CAD build for the part. Positions are in the model's coordinates, mm. A direction names the side the tool comes from. Round coordinates to 2 decimals unless told otherwise and drop trailing zeros. Write each loop counter-clockwise with the first axis right and the second up, starting at its lowest first coordinate (ties: lowest second). Pieces come first, ordered by that corner, then holes. Notation, with made-up numbers: (32, -10) - (36, -10) arc R30 cw to (36, 21) - close; hole circle Ø7 at (20.25, -36.75). An arc over 180 degrees is marked (long way). Put each result on its own line as item: value. Start each with the question number.
Item 1: Cut at B-B (z = 6). Give the cut face in (x, y).
Item 2: 3-axis set-ups, long thin cutter, end or side, ignore diameter. For faces 1 (the cylindrical face through (-2.579, -1.978, -0.493)), 2 (the flat face through (0, 0, -11)), 3 (the cylindrical face through (-0.325, -34.86, 4.536)), 4 (the flat face through (2, -2, 16)), 5 (the flat face through (0, -45, 6)): which of +Z, -Z, +X, -X, +Y, -Y reach the whole face in a straight line?
Item 3: Cut at C-C (y = 1.5). Give the cut face in (x, z).
Item 4: Cut at D-D (z = 2.5). Give the cut face in (x, y).
Item 5: Pin check, flat tips, straight feed: pin 1 Ø4 at (x, y) = (0.5, -16.5) entering from -Z; pin 2 Ø6 at (x, y) = (-1.5, -7) entering from +Z; pin 3 Ø12 at (x, y) = (-10, -8) entering from -Z; pin 4 Ø1.5 at (y, z) = (-15, 0) entering from +X. Stop position of each tip, or through.
Item 6: Cut at A-A (x = 0). Give the cut face in (y, z).
Item 7: Drill centre lines: line 1 (Z direction, x = 9, y = -2.5); line 2 (Y direction, x = -1.5, z = 22.5); line 3 (Z direction, x = 0.5, y = -39). Where is each one in solid material? Low to high. Write a range as from..to.
```python
from build123d import *

# Parameters (mm, degrees)
SKETCH_R     = 12.7
PAD_DEPTH    = 13
SKETCH001_R  = 5
PAD001_DEPTH = 3
SKETCH002_R  = 2.5
PAD002_DEPTH = 8
SKETCH003_R  = 3.25
PAD003_DEPTH = 1
SKETCH004_R  = 2.5
PAD004_DEPTH = 10
SKETCH005_R  = 2
PAD005_DEPTH = 25
SKETCH006_R  = 1.5
PAD006_DEPTH = 20


with BuildPart() as part:
    # Sketch → Pad (new body)
    with BuildSketch(Plane.XY):
        Circle(SKETCH_R)
    extrude(amount=PAD_DEPTH)

    # Sketch001 (on Face3 of Pad) → Pad001 (join)
    with BuildSketch(Plane.XY.offset(13)):
        Circle(SKETCH001_R)
    extrude(amount=PAD001_DEPTH)

    # Sketch002 (on Face5 of Pad001) → Pad002 (join)
    with BuildSketch(Plane.XY.offset(16)):
        Circle(SKETCH002_R)
    extrude(amount=PAD002_DEPTH)

    # Sketch003 → Pad003 (join)
    with BuildSketch(Plane.XY):
        Circle(SKETCH003_R)
    extrude(amount=-PAD003_DEPTH)

    # Sketch004 (on Face6 of Pad003) → Pad004 (join)
    with BuildSketch(Plane(origin=(0, 0, -1), x_dir=(1, 0, 0), z_dir=(0, 0, -1))):
        Circle(SKETCH004_R)
    extrude(amount=PAD004_DEPTH)

    # Sketch005 → Pad005 (join)
    with BuildSketch(Plane.XZ):
        with Locations((0, 6)):
            Circle(SKETCH005_R)
    extrude(amount=PAD005_DEPTH)

    # Sketch006 (on Face7 of Pad005) → Pad006 (join)
    with BuildSketch(Plane.XZ.offset(25)):
        with Locations((0, 6)):
            Circle(SKETCH006_R)
    extrude(amount=PAD006_DEPTH)


solid = part.part
```
Output values:
1. outline: (-2, -25) - (-1.5, -25) - (-1.5, -45) - (1.5, -45) - (1.5, -25) - (2, -25) - (2, -12.54) arc R12.7 ccw (long way) to (-2, -12.54) - close
2. face 1: -Z
2. face 2: -Z, +X, -X, +Y, -Y
2. face 3: -Y
2. face 4: +Z
2. face 5: +Z, -Z, +X, -X, -Y
3. outline: (-12.61, 0) - (-2.88, 0) - (-2.88, -1) - (-2, -1) - (-2, -11) - (2, -11) - (2, -1) - (2.88, -1) - (2.88, 0) - (12.61, 0) - (12.61, 13) - (4.77, 13) - (4.77, 16) - (2, 16) - (2, 24) - (-2, 24) - (-2, 16) - (-4.77, 16) - (-4.77, 13) - (-12.61, 13) - close
4. outline: circle Ø25.4 at (0, 0)
5. pin 1: z = 4
5. pin 2: z = 16
5. pin 3: z = 0
5. pin 4: through
6. outline: (-45, 4.5) - (-25, 4.5) - (-25, 4) - (-12.7, 4) - (-12.7, 0) - (-3.25, 0) - (-3.25, -1) - (-2.5, -1) - (-2.5, -11) - (2.5, -11) - (2.5, -1) - (3.25, -1) - (3.25, 0) - (12.7, 0) - (12.7, 13) - (5, 13) - (5, 16) - (2.5, 16) - (2.5, 24) - (-2.5, 24) - (-2.5, 16) - (-5, 16) - (-5, 13) - (-12.7, 13) - (-12.7, 8) - (-25, 8) - (-25, 7.5) - (-45, 7.5) - close
7. line 1: 0..13
7. line 2: -2..2
7. line 3: 4.59..7.41
